Source: CAD feature listing. Evaluate the final solid. Frame: model axes, mm. Give positions to 0.01 mm unless a question says otherwise; leave off trailing zeros. Order: outer loops, then holes, each group sorted by start corner. A loop starts at its lowest first (then second) coordinate and runs counter-clockwise, first axis right, second up.
1) Section C-C, the plane y = -24.5. Return loops of the section in (x, z), plus the area to 3 significant figures.
2) Section A-A, the plane x = -1.5. Return loops of the section in (y, z).
3) Section D-D, the plane y = -14.5. Return loops of the section in (x, z), plus the area to 3 significant figures.
4) Section B-B, the plane z = 30.5. Return loops of the section in (x, y), plus the area to 3 significant figures.
5) First-contact query: P1, Ø5, axis at y = -4.5, z = -5.5, coming from the +X side; P2, Ø8, axis at x = -25, z = 41.5, coming from the -Y side; P3, Ø8, axis at x = -19.5, y = -21.5, coming from the +Z side. Flat tips, straight axial feed; report the tip coordinate or a pass-through.
6) Material intervals for line 1 (Y direction, x = -25.5, z = 4); line 2 (Z direction, x = -14, y = -11.5); line 3 (Z direction, x = -7, y = -31.5), sorted ascending.
7) Draft query along X for faces 1 (the face through (0.491, -28.433, 49.792)), 2 (the face through (7.5, -17.91, -22.77)), 3 (the face through (-16, 0, 21)), 4 (the face through (-17, -20.32, 23)). Return one class per face: released by +X, released by -X, zero draft, split by the parting line, or undercut.
```python
from build123d import *

# Parameters (mm, degrees)
F0_R      = 48.999034
F1_DEPTH  = 50.8
F1_FACE_R = 48.999034
F2_DEPTH  = 14.478
F3_R      = 31.768864
F4_DEPTH  = 16.002


with BuildPart() as f1:
    # F0 (on Front) → F1 (new body)
    with BuildSketch(Plane.XZ):
        with Locations((-15.113131, 20.701002)):
            Circle(F0_R)
    extrude(amount=F1_DEPTH)

    # F1_face (on face) → F2 (cut)
    with BuildSketch(Plane(origin=(-15.113131, -50.8, 20.701002), x_dir=(1, 0, 0), z_dir=(0, -1, 0))):
        Circle(F1_FACE_R)
    extrude(amount=-F2_DEPTH, mode=Mode.SUBTRACT)

    # F3 (on face) → F4 (cut)
    with BuildSketch(Plane.XZ.offset(36.322)):
        with Locations((-16.587488, 23.004033)):
            Circle(F3_R)
    extrude(amount=-F4_DEPTH, mode=Mode.SUBTRACT)


solid = f1.part
```
From the geometry:
1. outline: circle Ø98 at (-15.11, 20.7); hole circle Ø63.54 at (-16.59, 23)
1. area: 4,370 mm2
2. outline: (-36.32, -26.37) - (0, -26.37) - (0, 67.77) - (-36.32, 67.77) - (-36.32, 50.96) - (-20.32, 50.96) - (-20.32, -4.95) - (-36.32, -4.95) - close
3. outline: circle Ø98 at (-15.11, 20.7)
3. area: 7,540 mm2
4. outline: (-63.12, -36.32) - (-47.46, -36.32) - (-47.46, -20.32) - (14.28, -20.32) - (14.28, -36.32) - (32.9, -36.32) - (32.9, 0) - (-63.12, 0) - close
4. area: 2,500 mm2
5. P1: stops at x = 27.77
5. P2: stops at y = -20.32
5. P3: stops at z = 69.7
6. line 1: y = -20.32 to 0
6. line 2: z = -28.29 to 69.69
6. line 3: z = -27.62 to -7.28, 53.29 to 69.02
7. face 1: undercut
7. face 2: split by the parting line
7. face 3: zero draft
7. face 4: undercut
